```python
from build123d import *

# Parameters (mm, degrees)
F0_W     = 200
F0_H     = 200
F1_DEPTH = 2.54
F2_R     = 12.7
F4_DEPTH = 2.541
F5_R     = 2.53999


# Not quite as in the source:
# - a fillet or chamfer is up to 0.001 mm smaller than in the source, because OpenCascade refuses the exact size


with BuildPart() as f1:
    # F0 (on Top) → F1 (new body)
    with BuildSketch(Plane.XY):
        with Locations((100, 100)):
            Rectangle(F0_W, F0_H)
    extrude(amount=F1_DEPTH)

    # F2
    f2_edges = [f1.edges().sort_by_distance(p)[0] for p in [
        (200, 0, 1.27),
        (200, 200, 1.27),
    ]]
    fillet(f2_edges, radius=F2_R)

    # F3 (on face) → F4 (cut, through all)
    with BuildSketch(Plane.XY.offset(2.54)):
        with BuildLine():
            Line((6.35, 193.65), (6.35, 6.35))
            Line((6.35, 6.35), (187.3, 6.35))
            ThreePointArc((187.3, 6.35), (191.7901280605, 8.2098719395), (193.65, 12.7))
            Line((193.65, 12.7), (193.65, 187.3))
            ThreePointArc((193.65, 187.3), (191.7901280605, 191.7901280605), (187.3, 193.65))
            Line((187.3, 193.65), (6.35, 193.65))
        make_face()
    extrude(amount=-F4_DEPTH, mode=Mode.SUBTRACT)

    # F5 (radius 2.54 in the source; OpenCascade refuses exactly that, so slightly less here)
    f5_edges = [f1.edges().sort_by_distance(p)[0] for p in [
        (96.825, 193.65, 2.54),
        (6.35, 100, 2.54),
        (196.280256, 196.280256, 2.54),
        (0, 100, 2.54),
    ]]
    fillet(f5_edges, radius=F5_R)


solid = f1.part
```
Geometry check sheet. Reference: the model listing, model coordinates, mm. Coordinates: 2 decimals unless noted, no trailing zeros. Write each loop counter-clockwise with the first axis right and the second up, starting at its lowest first coordinate (ties: lowest second). Pieces come first, ordered by that corner, then holes. Notation, with made-up numbers: M 25,87.5 L 34,87.5 A10 cw 34,100.5 Z; hole C 75.25,61 d7. An arc over 180 degrees is marked long. One line per item, written item: value. Start each with the question number.
(1) Scan lines: line 1 along Y through (x, z) = (98, 0.1); line 2 along X through (y, z) = (33, 0.3); line 3 along Y through (x, z) = (46, 1.65). Record each from-to range of solid material in increasing order. Write a range as [from, to].
(2) Depth check by flat-ended pin: pin 1 (1 mm diameter, centred on x = 72.5, z = 1.5, fed in from -Y). Enter the tip coordinate at first touch or a pass-through.
(3) Sectioned sample at C-C, the plane z = 0.6. Enter the section's corners in (x, y).
Filled sheet:
1. line 1: [0, 6.35], [193.65, 200]
1. line 2: [0.02, 6.33], [193.67, 199.98]
1. line 3: [0.61, 5.74], [194.26, 199.39]
2. pin 1: y = 0.21
3. outline: M 0.07,0.07 L 187.3,0.07 A12.63 ccw 199.93,12.7 L 199.93,187.3 A12.63 ccw 187.3,199.93 L 0.07,199.93 Z; hole M 6.28,6.28 L 187.3,6.28 A6.42 ccw 193.72,12.7 L 193.72,187.3 A6.42 ccw 187.3,193.72 L 6.28,193.72 Z
